Verification items for the finished model (mm, model axes). Face numbers are marked on the shaded views. A direction names the side the tool comes from. Round coordinates to 2 decimals unless told otherwise and drop trailing zeros. Write each loop counter-clockwise with the first axis right and the second up, starting at its lowest first coordinate (ties: lowest second). Pieces come first, ordered by that corner, then holes. Notation, with made-up numbers: (-21.75, 21.5) - (13.25, 21.5) arc R15 ccw to (13.25, 47.5) - close; hole circle Ø10 at (73, -39). An arc over 180 degrees is marked (long way). Write each question's results on one line, items separated by ' | '.
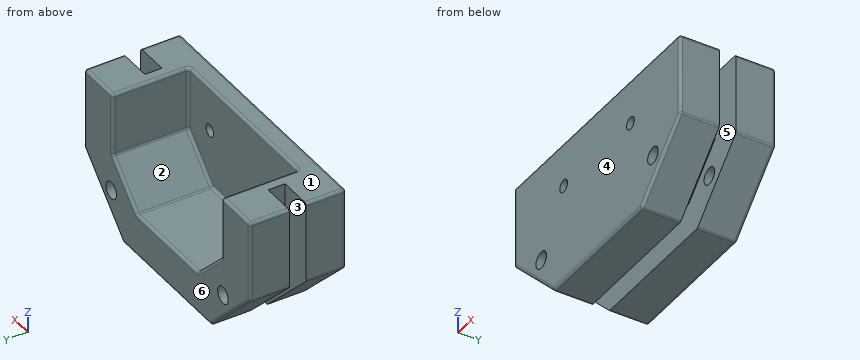
```python
from build123d import *

# Parameters (mm, degrees)
BOSS_EXTRUDE1_DEPTH      = 10
BOSS_EXTRUDE1_DEPTH_BACK = 7
BOSS_EXTRUDE4_START      = -7
BOSS_EXTRUDE4_DEPTH      = 3.5
FILLET1_R                = 0.5
CUT_EXTRUDE1_DEPTH       = 3
SKETCH2_R                = 1.5
CUT_EXTRUDE2_DEPTH       = 17
CUT_EXTRUDE3_START       = -3.5
SKETCH4_R                = 1.1
CUT_EXTRUDE3_DEPTH       = 3.5


with BuildPart() as part:
    # Sketch1 → Boss-Extrude1 (new body, two sides)
    with BuildSketch(Plane(origin=(0, 0, 0), x_dir=(1, 0, 0), z_dir=(0, 1, 0))) as boss_extrude1_sk:
        Polygon((21.473368866, -52.5), (29.473368866, -52.5), (29.473368866, -41.355058259), (36.328427125, -34.5), (53.671572875, -34.5), (60.526631134, -41.355058259), (60.526631134, -52.5), (68.526631134, -52.5), (68.526631134, -38.04134976), (57.485281374, -27), (32.514718626, -27), (21.473368866, -38.04134976), align=None)
    extrude(amount=BOSS_EXTRUDE1_DEPTH)
    extrude(boss_extrude1_sk.sketch, amount=-BOSS_EXTRUDE1_DEPTH_BACK)

    # Sketch1<5> → Boss-Extrude4 (add)
    with BuildSketch(Plane(origin=(0, 0, 0), x_dir=(1, 0, 0), z_dir=(0, 1, 0)).offset(BOSS_EXTRUDE4_START)):
        Polygon((60.526631134, -41.355058259), (60.526631134, -52.5), (29.473368866, -52.5), (29.473368866, -41.355058259), (36.328427125, -34.5), (53.671572875, -34.5), align=None)
    extrude(amount=BOSS_EXTRUDE4_DEPTH)

    # Fillet1
    fillet1_edges = [part.edges().sort_by_distance(p)[0] for p in [
        (45, -7, 52.5),
        (68.526631134, -7, 45.27067488),
        (63.005956254, -7, 32.52067488),
        (21.473368866, 1.5, 52.5),
        (21.473368866, 1.5, 38.04134976),
        (32.514718626, 1.5, 27),
        (57.485281374, 1.5, 27),
        (68.526631134, 1.5, 38.04134976),
        (68.526631134, 1.5, 52.5),
        (45, -7, 27),
        (26.994043746, -7, 32.52067488),
        (68.526631134, 10, 45.27067488),
        (63.005956254, 10, 32.52067488),
        (45, 10, 27),
        (26.994043746, 10, 32.52067488),
        (21.473368866, 10, 45.27067488),
        (25.473368866, 10, 52.5),
        (21.473368866, -7, 45.27067488),
        (60.526631134, 10, 46.927529129),
        (64.526631134, 10, 52.5),
        (29.473368866, 10, 46.927529129),
        (32.900897995, 10, 37.927529129),
        (45, 10, 34.5),
        (57.099102005, 10, 37.927529129),
        (60.526631134, 3.25, 52.5),
        (29.473368866, 3.25, 52.5),
        (29.473368866, 3.25, 41.355058259),
        (36.328427125, 3.25, 34.5),
        (53.671572875, 3.25, 34.5),
        (60.526631134, 3.25, 41.355058259),
        (45, -3.5, 52.5),
        (32.900897995, -3.5, 37.927529129),
        (29.473368866, -3.5, 46.927529129),
        (60.526631134, -3.5, 46.927529129),
        (57.099102005, -3.5, 37.927529129),
        (45, -3.5, 34.5),
    ]]
    fillet(fillet1_edges, radius=FILLET1_R)

    # Sketch1<3> → Cut-Extrude1 (cut)
    with BuildSketch(Plane(origin=(0, 0, 0), x_dir=(1, 0, 0), z_dir=(0, 1, 0))):
        Polygon((21.473368866, -52.5), (27.473368866, -52.5), (27.473368866, -40.526631134), (35, -33), (55, -33), (62.526631134, -40.526631134), (62.526631134, -52.5), (68.526631134, -52.5), (68.526631134, -38.04134976), (57.485281374, -27), (32.514718626, -27), (21.473368866, -38.04134976), align=None)
    extrude(amount=CUT_EXTRUDE1_DEPTH, mode=Mode.SUBTRACT)

    # Sketch2 → Cut-Extrude2 (cut)
    with BuildSketch(Plane(origin=(0, 10, 0), x_dir=(1, 0, 0), z_dir=(0, 1, 0))):
        with Locations((29.11536409, -34.641995223)):
            Circle(SKETCH2_R)
        with Locations((60.88463591, -34.641995223)):
            Circle(SKETCH2_R)
    extrude(amount=-CUT_EXTRUDE2_DEPTH, mode=Mode.SUBTRACT)

    # Sketch4 → Cut-Extrude3 (cut)
    with BuildSketch(Plane(origin=(0, 0, 0), x_dir=(1, 0, 0), z_dir=(0, 1, 0)).offset(CUT_EXTRUDE3_START)):
        with Locations((35.5, -44.5)):
            Circle(SKETCH4_R)
        with Locations((54.5, -44.5)):
            Circle(SKETCH4_R)
    extrude(amount=-CUT_EXTRUDE3_DEPTH, mode=Mode.SUBTRACT)


solid = part.part
```
(1) Thickness scan on L1, parallel to X at y = -5.9, z = 44.5; L2, parallel to X at y = 8, z = 50.5; L3, parallel to Y at x = 59, z = 35.25. Record the ranges inside material, lowest first.
Answer:
L1: 21.47 to 34.4, 36.6 to 53.4, 55.6 to 68.53 | L2: 21.47 to 29.47, 60.53 to 68.53 | L3: -7 to 0, 3 to 10
(2) Go/stop test with flat-tipped pins: pin 1 Ø0.9 at (y, z) = (1.5, 48.5) entering from +X; pin 2 Ø5 at (x, z) = (58.5, 45) entering from +Y; pin 3 Ø3 at (y, z) = (-4.5, 35) entering from -X; pin 4 Ø1.5 at (y, z) = (2, 46.5) entering from -X. Record where each tip stops, or that it passes through.
Answer:
pin 1: x = 62.53 | pin 2: y = 10 | pin 3: x = 23.01 | pin 4: x = 27.47
(3) Mould release check, pull along Y, two halves, no side actions. Record for the marked faces 4, 5 and 6: released by +Y, released by -Y, zero draft, split by the parting line, or undercut.
Answer:
face 4: released by -Y | face 5: undercut | face 6: released by +Y
(4) Section check C-C (x = 51). Record the cut outline in (y, z), plus the area to 3 significant figures.
Answer:
outline: (-7, 27.5) arc R0.5 ccw to (-6.5, 27) - (0, 27) - (0, 33) - (3, 33) - (3, 27) - (9.5, 27) arc R0.5 ccw to (10, 27.5) - (10, 34) arc R0.5 ccw to (9.5, 34.5) - (-3, 34.5) arc R0.5 cw to (-3.5, 35) - (-3.5, 52) arc R0.5 ccw to (-4, 52.5) - (-6.5, 52.5) arc R0.5 ccw to (-7, 52) - close | area: 172 mm2
(5) Section check A-A (z = 44.5). State how many separate pieces and enclosed holes the cut face has, plus the area to 3 significant figures.
Answer:
separate pieces: 3 | enclosed holes: 0 | area: 329 mm2
(6) Set-up check for the marked faces 1, 2 and 3: record each of +Z, -Z, +X, -X, +Y, -Y from which the full face is reachable in a straight line by a thin tool's end or side.
Answer:
face 1: +Z, +X, -X, +Y, -Y | face 2: +Z, +Y | face 3: -Z
(7) Section check B-B (y = -0.75). Record the cut outline in (x, z).
Answer:
outline: (21.47, 38.25) arc R0.5 ccw to (21.62, 37.89) - (32.37, 27.15) arc R0.5 ccw to (32.72, 27) - (57.28, 27) arc R0.5 ccw to (57.63, 27.15) - (68.38, 37.89) arc R0.5 ccw to (68.53, 38.25) - (68.53, 52) arc R0.5 ccw to (68.03, 52.5) - (61.03, 52.5) arc R0.5 ccw to (60.53, 52) - (60.53, 41.56) arc R0.5 cw to (60.38, 41.21) - (53.82, 34.65) arc R0.5 cw to (53.46, 34.5) - (36.54, 34.5) arc R0.5 cw to (36.18, 34.65) - (29.62, 41.21) arc R0.5 cw to (29.47, 41.56) - (29.47, 52) arc R0.5 ccw to (28.97, 52.5) - (21.97, 52.5) arc R0.5 ccw to (21.47, 52) - close; hole circle Ø3 at (29.12, 34.64); hole circle Ø3 at (60.88, 34.64)
